The listing builds one solid part. Answer for the finished solid, in the listing's coordinates (mm). A direction names the side the tool comes from. Coordinates: 2 decimals unless noted, no trailing zeros. Order: outer loops, then holes, each group sorted by start corner. A loop starts at its lowest first (then second) coordinate and runs counter-clockwise, first axis right, second up. Notation, with made-up numbers: (-2.5, 39.25) -> (47.5, 39.25) arc R24 ccw to (47.5, 75.25) -> close; hole circle Ø8 at (41, 25). An arc over 180 degrees is marked (long way). Return JSON: item names as keys, results as strings.
```python
from build123d import *

# Parameters (mm, degrees)
EXTRUDE_1_DEPTH     = 10
CUT_EXTRUDE_1_DEPTH = 3.2
SKETCH_3_R          = 2.5
CUT_EXTRUDE_2_DEPTH = 6
SKETCH_4_R          = 2
CUT_EXTRUDE_3_DEPTH = 6


with BuildPart() as part:
    # 草图1 → 凸台-拉伸1 (new body)
    with BuildSketch(Plane.XY):
        with BuildLine():
            Line((0, 13), (28, 13))
            Line((28, 13), (28, 23))
            Line((28, 23), (33, 23))
            Line((33, 23), (33, 10))
            Line((33, 10), (0, 10))
            ThreePointArc((0, 10), (-10, 0), (0, -10))
            Line((0, -10), (33, -10))
            Line((33, -10), (33, -23))
            Line((33, -23), (28, -23))
            Line((28, -23), (28, -13))
            Line((28, -13), (0, -13))
            ThreePointArc((0, -13), (-13, 0), (0, 13))
        make_face()
    extrude(amount=EXTRUDE_1_DEPTH)

    # 草图2 → 切除-拉伸1 (cut)
    with BuildSketch(Plane.ZY.offset(-28)):
        Polygon((8.5, 15.979274058), (8.5, 20.020725942), (5, 22.041451884), (1.5, 20.020725942), (1.5, 15.979274058), (5, 13.958548116), align=None)
    extrude(amount=-CUT_EXTRUDE_1_DEPTH, mode=Mode.SUBTRACT)

    # 草图3 → 切除-拉伸2 (cut, through all)
    with BuildSketch(Plane.ZY.offset(-28)):
        with Locations((5, 18)):
            Circle(SKETCH_3_R)
    extrude(amount=-CUT_EXTRUDE_2_DEPTH, mode=Mode.SUBTRACT)

    # 草图4 → 切除-拉伸3 (cut, through all)
    with BuildSketch(Plane.ZY.offset(-28)):
        with Locations((5, -18)):
            Circle(SKETCH_4_R)
    extrude(amount=-CUT_EXTRUDE_3_DEPTH, mode=Mode.SUBTRACT)


solid = part.part
```
Item 1: Determine the mould class of faces 1 (the flat face through (30, 18, 1.5)), 2 (the flat face through (28, -20.3, 4.9)), 3 (the flat face through (13.5, 10.3, 10)), 4 (the flat face through (29.578, 21.045, 3.274)) for opening direction Z: pulls with the +Z half, pulls with the -Z half, needs draft (parallel to the pull), parting line crosses it, or undercut.
Answer list:
{"face 1": "undercut", "face 2": "needs draft", "face 3": "pulls with the +Z half", "face 4": "undercut"}
Item 2: Which of the six approach directions +Z, -Z, +X, -X, +Y, -Y give full straight-line access (tool end or side, diameter ignored) to faces 5 (the flat face through (14, 13, 5)), 6 (the flat face through (16, -10, 5)), 7 (the flat face through (31.2, 15, 5))?
Answer list:
{"face 5": "+Z, -Z, -X, +Y", "face 6": "+Z, -Z, +X", "face 7": "-X"}
Item 3: The part is cut by section C-C on x = 4. Determine the outline of the cut face in (y, z).
Answer list:
{"outline": "(-13, 0) -> (-10, 0) -> (-10, 10) -> (-13, 10) -> close; (10, 0) -> (13, 0) -> (13, 10) -> (10, 10) -> close"}
Item 4: The part is cut by section D-D on y = 18. Determine the outline of the cut face in (x, z).
Answer list:
{"outline": "(28, 0) -> (33, 0) -> (33, 2.5) -> (31.2, 2.5) -> (31.2, 1.5) -> (28, 1.5) -> close; (28, 8.5) -> (31.2, 8.5) -> (31.2, 7.5) -> (33, 7.5) -> (33, 10) -> (28, 10) -> close"}
Item 5: The part is cut by section A-A on x = 30.5. Determine the outline of the cut face in (y, z), plus the area to 3 significant figures.
Answer list:
{"outline": "(-23, 0) -> (-10, 0) -> (-10, 10) -> (-23, 10) -> close; (10, 0) -> (23, 0) -> (23, 10) -> (10, 10) -> close; hole circle Ø4 at (-18, 5); hole (13.96, 5) -> (15.98, 1.5) -> (20.02, 1.5) -> (22.04, 5) -> (20.02, 8.5) -> (15.98, 8.5) -> close", "area": "205 mm2"}
Item 6: Flat-ended cylindrical pins translate along their axes: pin 1 (5 mm diameter, centred on x = 14.5, z = 3.5, fed in from +Y); pin 2 (3 mm diameter, centred on y = -20, z = 6.5, fed in from -X); pin 3 (2 mm diameter, centred on y = 19, z = 3.5, fed in from -X). Find the tip coordinate at first contact, or state that the pin passes through.
Answer list:
{"pin 1": "y = 13", "pin 2": "x = 28", "pin 3": "x = 31.2"}
Item 7: The part is cut by section B-B on y = -18. Determine the outline of the cut face in (x, z).
Answer list:
{"outline": "(28, 0) -> (33, 0) -> (33, 3) -> (28, 3) -> close; (28, 7) -> (33, 7) -> (33, 10) -> (28, 10) -> close"}
Item 8: Find the intervals of material crossed by probe 1 along Y at (x, z) = (32.2, 5); probe 2 along Y at (x, z) = (29.7, 5); probe 3 along Y at (x, z) = (12, 3.25), in increasing order.
Answer list:
{"probe 1": "-23 to -20, -16 to -10, 10 to 15.5, 20.5 to 23", "probe 2": "-23 to -20, -16 to -10, 10 to 13.96, 22.04 to 23", "probe 3": "-13 to -10, 10 to 13"}
